Work out the finished part from the listing and answer in its coordinate system (mm). Face numbers are marked on the shaded views. A direction names the side the tool comes from. Coordinates: 2 decimals unless noted, no trailing zeros. Order: outer loops, then holes, each group sorted by start corner. A loop starts at its lowest first (then second) coordinate and runs counter-clockwise, first axis right, second up.
1. A tool of negligible diameter and unlimited length cuts with its end or side. For the marked faces 4, 5 and 6, from which of +Z, -Z, +X, -X, +Y, -Y can it reach the whole face along a straight path? Write none if from no direction.
2. The part is cut by section C-C, the plane y = -7.75. Give the vertices of the cut face in (x, z).
3. The part is cut by section A-A, the plane y = -1.75. Give the vertices of the cut face in (x, z).
4. Determine the mould class of the marked faces 1, 2 and 3 for opening direction X: +X half, -X half, draft (parallel to the pull), parting line (faces both ways), or undercut.
5. Flat-ended cylindrical pins translate along their axes: pin 1 Ø6 at (x, y) = (-9.5, -5) entering from -Z; pin 2 Ø3 at (x, z) = (4.5, -1) entering from -Y; pin 3 Ø1 at (y, z) = (-1.5, -2) entering from -X. Find the tip coordinate at first contact, or state that the pin passes through.
6. Find the intervals of material crossed by probe 1 along Y at (x, z) = (5, -7); probe 2 along X at (y, z) = (-4, 0.5); probe 3 along X at (y, z) = (-1.5, 2.25), in increasing order.
7. The part is cut by section B-B, the plane z = 0. Give the vertices of the cut face in (x, y), then the cut area to 3 significant figures.
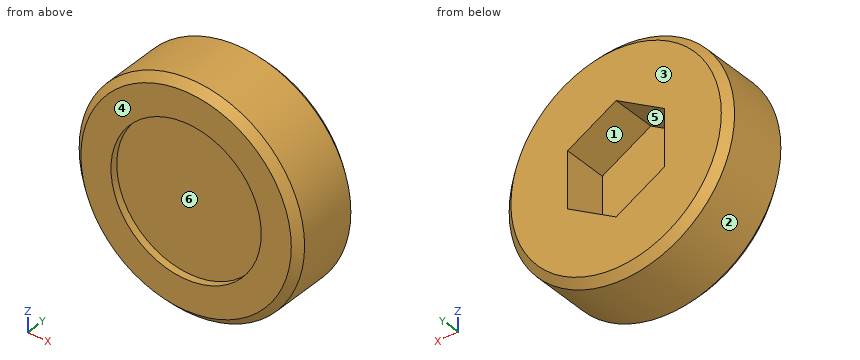
```python
from build123d import *

# Parameters (mm, degrees)
SKETCH_R        = 15
PAD_DEPTH       = 10
POCKET_DEPTH    = 6
SKETCH002_R     = 10
POCKET001_DEPTH = 1
CHAMFER_SIZE    = 1


with BuildPart() as part:
    # Sketch → Pad (new body)
    with BuildSketch(Plane.XZ):
        Circle(SKETCH_R)
    extrude(amount=PAD_DEPTH)

    # Sketch001 → Pocket (cut)
    with BuildSketch(Plane.XZ):
        Polygon((6.45, -3.723909), (6.45, 3.723909), (0, 7.447818), (-6.45, 3.723909), (-6.45, -3.723909), (0, -7.447818), align=None)
    extrude(amount=POCKET_DEPTH, mode=Mode.SUBTRACT)

    # Sketch002 (on Face3 of Pocket) → Pocket001 (cut)
    with BuildSketch(Plane.XZ.offset(10)):
        Circle(SKETCH002_R)
    extrude(amount=-POCKET001_DEPTH, mode=Mode.SUBTRACT)

    # Chamfer
    chamfer_edges = [part.edges().sort_by_distance(p)[0] for p in [
        (-15, -10, 0),
        (-15, 0, 0),
    ]]
    chamfer(chamfer_edges, length=CHAMFER_SIZE)


solid = part.part
```
Geometry says:
1. face 4: +Z, -Z, +X, -X, -Y
1. face 5: +Y
1. face 6: -Y
2. outline: circle Ø30 at (0, 0)
3. outline: circle Ø30 at (0, 0); hole (-6.45, -3.72) - (0, -7.45) - (6.45, -3.72) - (6.45, 3.72) - (0, 7.45) - (-6.45, 3.72) - close
4. face 1: undercut
4. face 2: parting line
4. face 3: draft
5. pin 1: stops at z = -13.52
5. pin 2: stops at y = -9
5. pin 3: stops at x = -14.92
6. probe 1: y = -9 to 0
6. probe 2: x = -14.99 to -6.45, 6.45 to 14.99
6. probe 3: x = -14.83 to -6.45, 6.45 to 14.83
7. outline: (-15, -9) - (-14, -10) - (-10, -10) - (-10, -9) - (10, -9) - (10, -10) - (14, -10) - (15, -9) - (15, -1) - (14, 0) - (6.45, 0) - (6.45, -6) - (-6.45, -6) - (-6.45, 0) - (-14, 0) - (-15, -1) - close
7. area: 201 mm2
